Could you check a few things on this drawing? It's one solid part, dimensions in mm from its lowest x, y, z. A direction names the side the tool comes from. Round coordinates to 2 decimals unless told otherwise and drop trailing zeros. Write each loop counter-clockwise with the first axis right and the second up, starting at its lowest first coordinate (ties: lowest second). Pieces come first, ordered by that corner, then holes. Notation, with made-up numbers: (-32.75, 86) -> (0.25, 86) arc R27 ccw to (0.25, 103) -> close; hole circle Ø4 at (64, 48.25). An arc over 180 degrees is marked (long way). Put each result on its own line as item: value. Start each with the question number.
1) I want a section at B-B, the plane y = 6.5. List the corners of the cut face in (x, z) for me (1 decimal).
2) I want a section at A-A, the plane x = 17.25. List the corners of the cut face in (y, z) for me.
3) Which directions (+Z, -Z, +X, -X, +Y, -Y) give clear straight access to the entire face, cutting with the end or side of a thin tool? Please do the marked faces 1 and 2.
4) Will these pins go through, and if not, where does the flat tip stop? P1, Ø6, axis at x = 7.5, y = 12.5, coming from the +Z side; P2, Ø5, axis at x = 15, z = 15, coming from the -Y side; P3, Ø5, axis at x = 5.5, y = 13, coming from the +Z side; P4, Ø1.5, axis at x = 2, z = 3, coming from the -Y side.
5) If I drill on line 1 along Y through (x, z) = (15, 13); line 2 along X through (y, z) = (13, 8.5) (1 decimal); line 3 along X through (y, z) = (20.75, 1), over which ranges is the centre line in solid material (lowest first)? Write a range as [from, to].
6) I want a section at C-C, the plane x = 3. List the corners of the cut face in (y, z) for me.
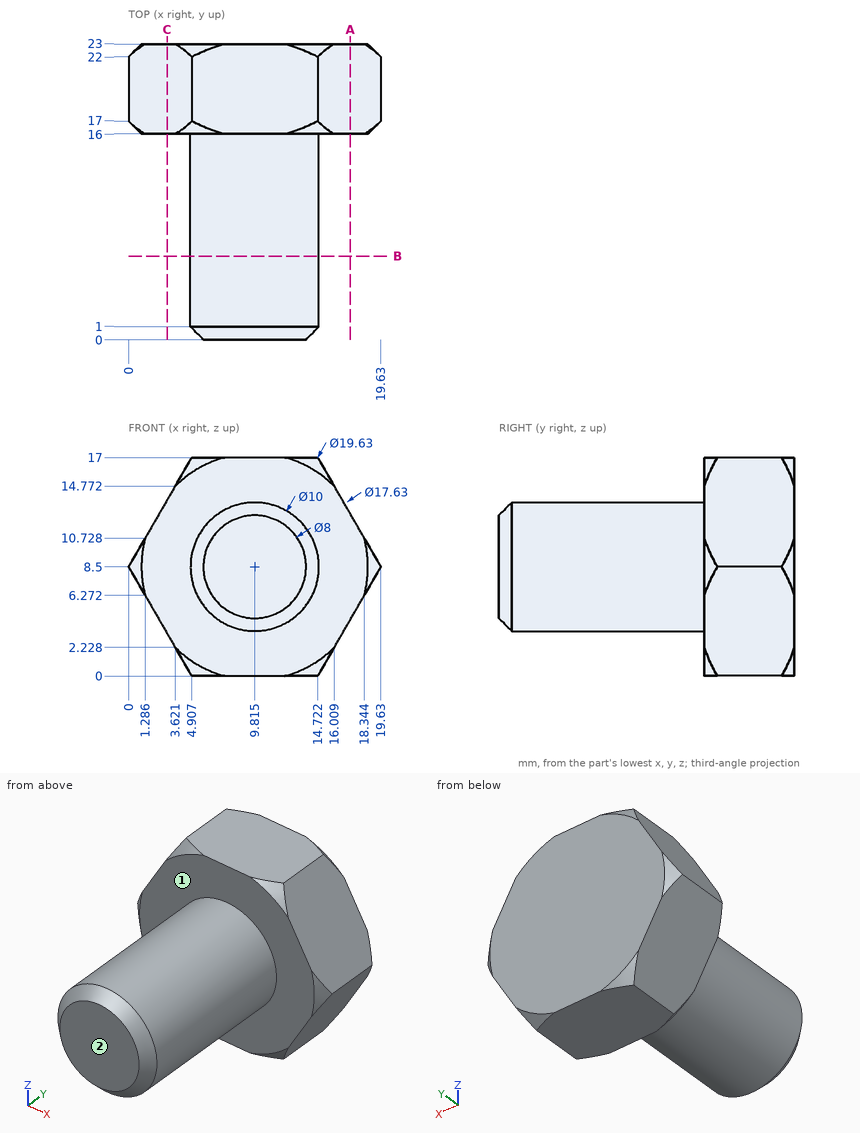
Findings:
1. outline: circle Ø10 at (9.8, 8.5)
2. outline: (16, 4.38) -> (23, 4.38) -> (23, 12.62) -> (16, 12.62) -> close
3. face 1: -Y
3. face 2: +Z, -Z, +X, -X, -Y
4. P1: stops at z = 13.5
4. P2: stops at y = 16
4. P3: stops at z = 13.16
4. P4: passes through
5. line 1: y = [16, 23]
5. line 2: x = [4.8, 14.8]
5. line 3: x = [4.33, 15.3]
6. outline: (16, 3.3) -> (23, 3.3) -> (23, 13.7) -> (16, 13.7) -> close
